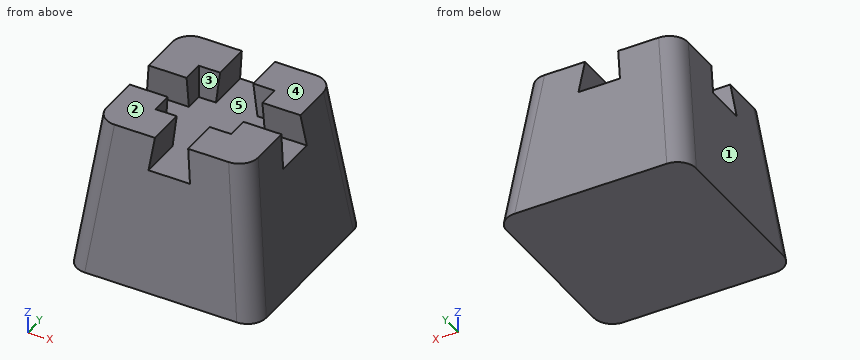
```python
from build123d import *

# Parameters (mm, degrees)
F0_W     = 254
F0_H     = 254
F1_DEPTH = 203.2
F1_TAPER = 7.125
F2_R     = 25.4
F4_DEPTH = 44.45
F4_TAPER = -7.125
F5_W     = 101.6
F5_H     = 101.6
F6_DEPTH = 44.45


with BuildPart() as f1:
    # F0 (on Top) → F1 (new body)
    with BuildSketch(Plane.XY):
        with Locations((-0.4685800523, 11.0039802372)):
            Rectangle(F0_W, F0_H)
    extrude(amount=F1_DEPTH, taper=F1_TAPER)

    # F2
    f2_edges = [f1.edges().sort_by_distance(p)[0] for p in [
        (-114.768609, -103.296049, 101.6),
        (113.831449, -103.296049, 101.6),
        (113.831449, 125.304009, 101.600004),
        (-114.768609, 125.30401, 101.6),
    ]]
    fillet(f2_edges, radius=F2_R)

    # F3 (on face) → F4 (cut)
    with BuildSketch(Plane.XY.offset(203.2)):
        Polygon((-22.6936389397, 33.2289213498), (-102.0686389397, 33.2289213498), (-102.0686389397, -11.2210786502), (-22.6936389397, -11.2210786502), (-22.6936389397, -90.5960786502), (21.7563610603, -90.5960786502), (21.7563610603, -11.2210786502), (101.1314788352, -11.2210786502), (101.1314788352, 33.2289213498), (21.7563610603, 33.2289213498), (21.7563610603, 112.6040391247), (-22.6936389397, 112.6040391247), align=None)
    extrude(amount=-F4_DEPTH, taper=F4_TAPER, mode=Mode.SUBTRACT)

    # F5 (on face) → F6 (cut)
    with BuildSketch(Plane.XY.offset(203.2)):
        with Locations((-0.4685211648, 11.0039213498)):
            Rectangle(F5_W, F5_H)
    extrude(amount=-F6_DEPTH, mode=Mode.SUBTRACT)


solid = f1.part
```
Work out the finished part from the listing and answer in its coordinate system (mm). Face numbers are marked on the shaded views. A direction names the side the tool comes from. Coordinates: 2 decimals unless noted, no trailing zeros. Loops run counter-clockwise (first coordinate to the right, second up) from the corner with the lowest first, then second, coordinate; pieces in that order, holes last. Notation, with made-up numbers: (85, 80) - (141, 80) arc R25 ccw to (141, 117) - close; hole circle Ø10 at (81.5, 30). An arc over 180 degrees is marked (long way). Use a Markdown table: item, result.
Item 1: Find section C-C, the plane x = 4. Determine the outline of the cut face in (y, z).
Evaluation:
| item | result |
|---|---|
| outline | (-116, 0) - (138, 0) - (118.16, 158.75) - (-96.15, 158.75) - close |
Item 2: Find section A-A, the plane x = -32.5. Determine the outline of the cut face in (y, z), and give its area (3 significant figures).
Evaluation:
| item | result |
|---|---|
| outline | (-116, 0) - (138, 0) - (112.6, 203.2) - (61.8, 203.2) - (61.8, 158.75) - (-39.8, 158.75) - (-39.8, 203.2) - (-90.6, 203.2) - close |
| area | 41,900 mm2 |
Item 3: Consider probe 1 along Y at (x, z) = (94.5, 191); probe 2 along Z at (x, y) = (60, 20); probe 3 along X at (y, z) = (-50, 187). Determine where each line is inside the solid, lowest interval first. Write a range as from..to.
Evaluation:
| item | result |
|---|---|
| probe 1 | y = -85.53..-12.75, 34.75..107.53 |
| probe 2 | z = 0..158.75 |
| probe 3 | x = -104.09..-24.72, 23.78..103.16 |
Item 4: Given pin 1 Ø3 at (y, z) = (-2, 61.5) entering from +X; pin 2 Ø10 at (y, z) = (-70, 24) entering from -X; pin 3 Ø1.5 at (x, y) = (50, 2) entering from +Z, each flat-ended and moving along its own axis, determine where each tip first touches the part or whether it passes through.
Evaluation:
| item | result |
|---|---|
| pin 1 | stops at x = 119.03 |
| pin 2 | stops at x = -125.09 |
| pin 3 | stops at z = 158.75 |
Item 5: The mould has two halves that part along X. Classify the marked faces 1, 2 and 3: +X half, -X half, draft (parallel to the pull), parting line (faces both ways), or undercut.
Evaluation:
| item | result |
|---|---|
| face 1 | -X half |
| face 2 | draft |
| face 3 | undercut |
Item 6: Find section B-B, the plane z = 182.5. State how many separate pieces and enclosed holes the cut face has, and give its area (3 significant figures).
Evaluation:
| item | result |
|---|---|
| separate pieces | 4 |
| enclosed holes | 0 |
| area | 22,000 mm2 |
Item 7: For the marked faces 4 and 5, determine the directions among +Z, -Z, +X, -X, +Y, -Y from which every point of the face is accessible in a straight line to the end or side of a thin tool.
Evaluation:
| item | result |
|---|---|
| face 4 | +Z, +X, -X, +Y, -Y |
| face 5 | none |
